Drawing for the job (mm, zero at the part's lowest x, y, z). Coordinates: 2 decimals unless noted, no trailing zeros. Order: outer loops, then holes, each group sorted by start corner. A loop starts at its lowest first (then second) coordinate and runs counter-clockwise, first axis right, second up.
1) Wall check: L1, parallel to X at y = 0.8, z = 18; L2, parallel to X at y = 0.4, z = 13; L3, parallel to Z at x = 19.5, y = 1.3 (1 decimal). Give the ranges that are in metal, low to high.
2) Cut at C-C (y = 0.7). Give the number of separate pieces and of enclosed holes in the cut face.
3) Cut at A-A (x = 22.86). List the corners of the cut face in (y, z) (1 decimal), and give its area (3 significant figures).
4) Pin check, flat tips, straight feed: pin 1 Ø0.5 at (x, y) = (27.5, 1) entering from -Z; pin 2 Ø0.8 at (x, y) = (44.5, 0.5) entering from -Z. Stop position of each tip, or through.
5) Cut at B-B (z = 21). List the corners of the cut face in (x, y) (1 decimal).
6) Cut at D-D (z = 14). List the corners of the cut face in (x, y) (1 decimal).
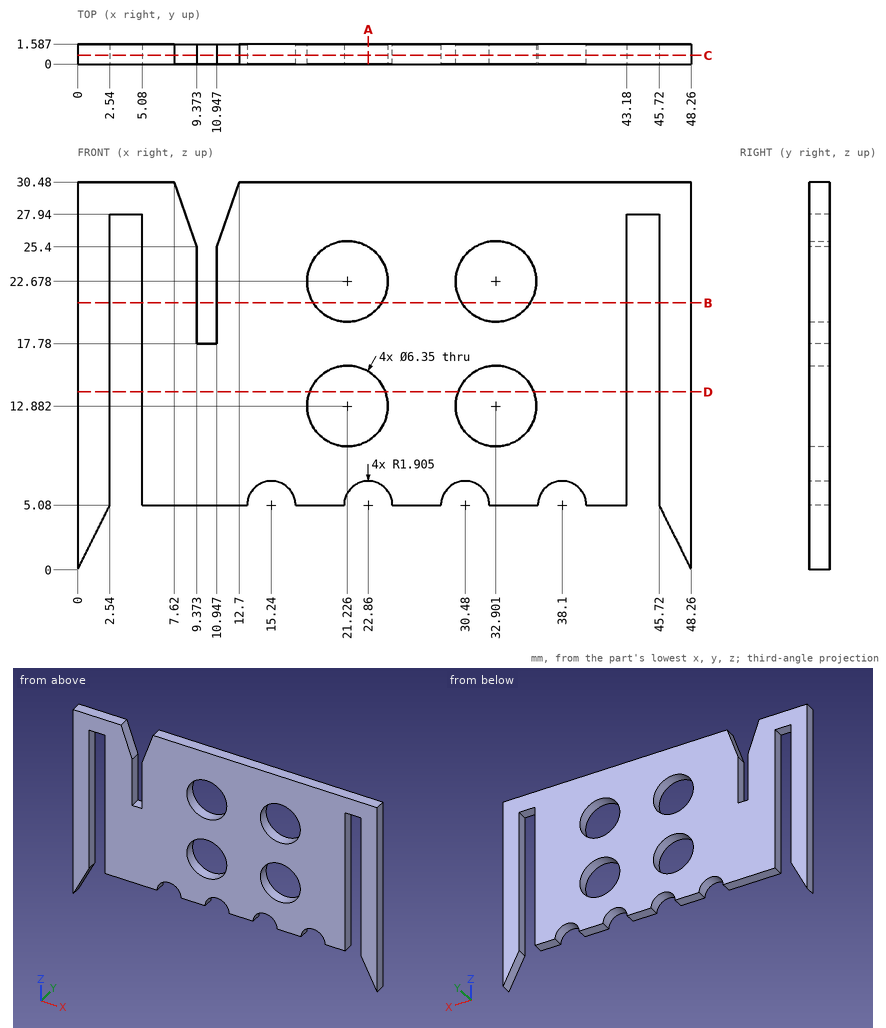
Geometry check:
1. L1: x = 0 to 2.54, 5.08 to 9.37, 10.95 to 43.18, 45.72 to 48.26
1. L2: x = 0 to 2.54, 5.08 to 18.05, 24.4 to 29.73, 36.07 to 43.18, 45.72 to 48.26
1. L3: z = 5.1 to 10.2, 15.5 to 20, 25.3 to 30.5
2. separate pieces: 1
2. enclosed holes: 4
3. outline: (0, 7) - (1.6, 7) - (1.6, 10.2) - (0, 10.2) - close; (0, 15.6) - (1.6, 15.6) - (1.6, 20) - (0, 20) - close; (0, 25.4) - (1.6, 25.4) - (1.6, 30.5) - (0, 30.5) - close
3. area: 20.0 mm2
4. pin 1: stops at z = 5.08
4. pin 2: stops at z = 27.94
5. outline: (0, 0) - (2.5, 0) - (2.5, 1.6) - (0, 1.6) - close; (5.1, 0) - (9.4, 0) - (9.4, 1.6) - (5.1, 1.6) - close; (10.9, 0) - (18.5, 0) - (18.5, 1.6) - (10.9, 1.6) - close; (23.9, 0) - (30.2, 0) - (30.2, 1.6) - (23.9, 1.6) - close; (35.6, 0) - (43.2, 0) - (43.2, 1.6) - (35.6, 1.6) - close; (45.7, 0) - (48.3, 0) - (48.3, 1.6) - (45.7, 1.6) - close
6. outline: (0, 0) - (2.5, 0) - (2.5, 1.6) - (0, 1.6) - close; (5.1, 0) - (18.3, 0) - (18.3, 1.6) - (5.1, 1.6) - close; (24.2, 0) - (29.9, 0) - (29.9, 1.6) - (24.2, 1.6) - close; (35.9, 0) - (43.2, 0) - (43.2, 1.6) - (35.9, 1.6) - close; (45.7, 0) - (48.3, 0) - (48.3, 1.6) - (45.7, 1.6) - close
